Geometry: final body of the model. Coordinates: model frame, mm. A direction names the side the tool comes from. Coordinates: 2 decimals unless noted, no trailing zeros. Write each loop counter-clockwise with the first axis right and the second up, starting at its lowest first coordinate (ties: lowest second). Pieces come first, ordered by that corner, then holes.
from build123d import *

# Parameters (mm, degrees)
SKETCH_1_R          = 50.5
EXTRUDE_1_DEPTH     = 2
SKETCH_2_R          = 11.25
SKETCH_2_R_2        = 2.1
CUT_EXTRUDE_1_DEPTH = 10
FILLET_1_R          = 3


with BuildPart() as part:
    # 草图1 → 凸台-拉伸1 (new body)
    with BuildSketch(Plane.XY):
        Circle(SKETCH_1_R)
    extrude(amount=EXTRUDE_1_DEPTH)

    # 草图2 → 切除-拉伸1 (cut)
    with BuildSketch(Plane.XY.offset(2)):
        with BuildLine():
            Line((-5, 22.706001409), (-5, 37.165171868))
            ThreePointArc((-5, 37.165171868), (-32.475952642, 18.75), (-34.685982974, -14.252458915))
            Line((-34.685982974, -14.252458915), (-22.163974039, -7.022873686))
            ThreePointArc((-22.163974039, -7.022873686), (-20.135090638, 11.625), (-5, 22.706001409))
        make_face()
        with BuildLine():
            ThreePointArc((37.5, 0), (28.228974477, 24.685522073), (5, 37.165171868))
            Line((5, 37.165171868), (5, 22.706001409))
            ThreePointArc((5, 22.706001409), (18.121982507, 14.565584437), (23.25, 0))
            ThreePointArc((23.25, 0), (22.976889437, -3.55317489), (22.163974039, -7.022873686))
            Line((22.163974039, -7.022873686), (34.685982974, -14.252458915))
            ThreePointArc((34.685982974, -14.252458915), (36.789770056, -7.263801982), (37.5, 0))
        make_face()
        with BuildLine():
            Line((-17.163974039, -15.683127724), (-29.685982974, -22.912712953))
            ThreePointArc((-29.685982974, -22.912712953), (0, -37.5), (29.685982974, -22.912712953))
            Line((29.685982974, -22.912712953), (17.163974039, -15.683127724))
            ThreePointArc((17.163974039, -15.683127724), (0, -23.25), (-17.163974039, -15.683127724))
        make_face()
        Circle(SKETCH_2_R)
        with Locations((-14.938938215, -8.625)):
            Circle(SKETCH_2_R_2)
        with Locations((-14.938938215, 8.625)):
            Circle(SKETCH_2_R_2)
        with Locations((0, 17.25)):
            Circle(SKETCH_2_R_2)
        with Locations((14.938938215, 8.625)):
            Circle(SKETCH_2_R_2)
        with Locations((14.938938215, -8.625)):
            Circle(SKETCH_2_R_2)
        with Locations((0, -17.25)):
            Circle(SKETCH_2_R_2)
    extrude(amount=-CUT_EXTRUDE_1_DEPTH, mode=Mode.SUBTRACT)

    # 圆角1
    fillet_1_edges = [part.edges().sort_by_distance(p)[0] for p in [
        (34.685982974, -14.252458915, 1),
        (22.163974039, -7.022873686, 1),
        (5, 22.706001409, 1),
        (5, 37.165171868, 1),
        (-29.685982974, -22.912712953, 1),
        (-17.163974039, -15.683127724, 1),
        (17.163974039, -15.683127724, 1),
        (29.685982974, -22.912712953, 1),
        (-5, 37.165171868, 1),
        (-5, 22.706001409, 1),
        (-22.163974039, -7.022873686, 1),
        (-34.685982974, -14.252458915, 1),
    ]]
    fillet(fillet_1_edges, radius=FILLET_1_R)


solid = part.part
Item 1: Section D-D, the plane z = 0.85. State how many separate pieces and enclosed holes the cut face has, plus the area to 3 significant figures.
Derived:
separate pieces: 1
enclosed holes: 10
area: 5,270 mm2
Item 2: Section B-B, the plane y = 17.25. Output: boundary loops of the cut face in (x, z).
Derived:
outline: (-47.46, 0) - (-33.3, 0) - (-33.3, 2) - (-47.46, 2) - close; (-15.59, 0) - (-2.1, 0) - (-2.1, 2) - (-15.59, 2) - close; (2.1, 0) - (15.59, 0) - (15.59, 2) - (2.1, 2) - close; (33.3, 0) - (47.46, 0) - (47.46, 2) - (33.3, 2) - close
Item 3: Material intervals for probe 1 along Y at (x, z) = (0, 1.4); probe 2 along Y at (x, z) = (19, 0.7); probe 3 along Y at (x, z) = (-3.5, 1.1), sorted ascending.
Derived:
probe 1: y = -50.5 to -37.5, -23.25 to -19.35, -15.15 to -11.25, 11.25 to 15.15, 19.35 to 50.5
probe 2: y = -46.79 to -32.33, -16.75 to 13.4, 32.33 to 46.79
probe 3: y = -50.38 to -37.34, -22.99 to -10.69, 10.69 to 50.38
Item 4: Section A-A, the plane x = 0. Output: boundary loops of the cut face in (y, z), plus the area to 3 significant figures.
Derived:
outline: (-50.5, 0) - (-37.5, 0) - (-37.5, 2) - (-50.5, 2) - close; (-23.25, 0) - (-19.35, 0) - (-19.35, 2) - (-23.25, 2) - close; (-15.15, 0) - (-11.25, 0) - (-11.25, 2) - (-15.15, 2) - close; (11.25, 0) - (15.15, 0) - (15.15, 2) - (11.25, 2) - close; (19.35, 0) - (50.5, 0) - (50.5, 2) - (19.35, 2) - close
area: 112 mm2
Item 5: Section C-C, the plane y = -35. Output: boundary loops of the cut face in (x, z).
Derived:
outline: (-36.4, 0) - (-13.46, 0) - (-13.46, 2) - (-36.4, 2) - close; (13.46, 0) - (36.4, 0) - (36.4, 2) - (13.46, 2) - close
Item 6: Set-up query: faces 5 (the cylindrical face through (-6.11, 35.89, 0.99)), 6 (the flat face through (-1, 12, 2)). Return all of +Z, -Z, +X, -X, +Y, -Y with unobstructed straight access to the full face (end or side cutting, diameter ignored); none if empty.
Derived:
face 5: +Z, -Z
face 6: +Z, +X, -X, +Y, -Y
Item 7: Pin query (flat end, axial travel): pin 1 (4 mm diameter, centred on x = -14.94, y = 8.62, fed in from +Z); pin 2 (1 mm diameter, centred on x = -14, z = 0.5, fed in from +Y); pin 3 (1 mm diameter, centred on y = 30.5, z = 1, fed in from +X); pin 4 (1 mm diameter, centred on y = 28, z = 0.5, fed in from -X). Return the tip coordinate at first contact, or that it passes through.
Derived:
pin 1: passes through
pin 2: stops at y = 48.66
pin 3: stops at x = 40.62
pin 4: stops at x = -42.36
Item 8: Pull-direction query (X, two-part tool) for faces 1 (the cylindrical face through (5.19, -9.98, 1.01)), 2 (the cylindrical face through (-32.26, 19.12, 1.01)), 3 (the flat face through (-1, 12, 0)), 4 (the cylindrical face through (-10.95, -49.3, 0.99)); classes: released by +X, released by -X, zero draft, split by the parting line, or undercut.
Derived:
face 1: undercut
face 2: undercut
face 3: zero draft
face 4: split by the parting line
